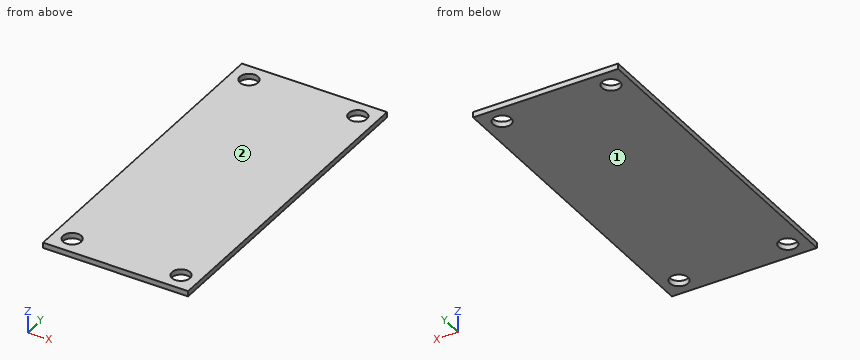
from build123d import *

# Parameters (mm, degrees)
SKETCH1_W           = 40
SKETCH1_H           = 41
BOSS_EXTRUDE1_DEPTH = 1.5
SKETCH2_R           = 2.5
CUT_EXTRUDE1_DEPTH  = 270.746640387


with BuildPart() as part:
    # Sketch1 → Boss-Extrude1 (new body)
    with BuildSketch(Plane.XY):
        Polygon((10, 269), (-10, 269), (-20, 269), (-20, 261), (-20, 220), (20, 220), (20, 261), (20, 269), align=None)
        with Locations((0, 199.5)):
            Rectangle(SKETCH1_W, SKETCH1_H)
    extrude(amount=BOSS_EXTRUDE1_DEPTH)

    # Sketch2 → Cut-Extrude1 (cut, through all)
    with BuildSketch(Plane.XY.offset(1.5)):
        with Locations((15, 264)):
            Circle(SKETCH2_R)
        with Locations(Location((15, 184, 0), (0, 0, 180))):
            Circle(SKETCH2_R)
        with Locations((-15, 184)):
            Circle(SKETCH2_R)
        with Locations(Location((-15, 264, 0), (0, 0, 180))):
            Circle(SKETCH2_R)
    extrude(amount=-CUT_EXTRUDE1_DEPTH, mode=Mode.SUBTRACT)


solid = part.part
The listing builds one solid part. Answer for the finished solid, in the listing's coordinates (mm). Face numbers are marked on the shaded views. Coordinates: 2 decimals unless noted, no trailing zeros. Order: outer loops, then holes, each group sorted by start corner. A loop starts at its lowest first (then second) coordinate and runs counter-clockwise, first axis right, second up.
Q1. For a pull along Z with two mould halves and no side action, classify the marked faces 1 and 2 as pulls with the +Z half, pulls with the -Z half, needs draft (parallel to the pull), parting line crosses it, or undercut.
Q2. A cutting plane is placed at A-A, the plane x = 15. Write down the section's boundary in (y, z).
Q3. A cutting plane is placed at C-C, the plane z = 0.75. Write down the section's boundary in (x, y), and give its area (3 significant figures).
Q4. Consider line 1 (Y direction, x = -15, z = 1); line 2 (X direction, y = 184, z = 0.45); line 3 (X direction, y = 262.5, z = 0.2). Determine where each line is inside the solid, lowest interval first.
Q5. A cutting plane is placed at B-B, the plane y = 184. Write down the section's boundary in (x, z), and give its area (3 significant figures).
Q6. Given P1, Ø6.5, axis at x = -15, y = 184, coming from the +Z side, flat-ended and moving along its own axis, determine where the tip first touches the part or whether it passes through.
Answers follow:
1. face 1: pulls with the -Z half
1. face 2: pulls with the +Z half
2. outline: (179, 0) - (181.5, 0) - (181.5, 1.5) - (179, 1.5) - close; (186.5, 0) - (261.5, 0) - (261.5, 1.5) - (186.5, 1.5) - close; (266.5, 0) - (269, 0) - (269, 1.5) - (266.5, 1.5) - close
3. outline: (-20, 179) - (20, 179) - (20, 269) - (-20, 269) - close; hole circle Ø5 at (-15, 184); hole circle Ø5 at (-15, 264); hole circle Ø5 at (15, 184); hole circle Ø5 at (15, 264)
3. area: 3,520 mm2
4. line 1: y = 179 to 181.5, 186.5 to 261.5, 266.5 to 269
4. line 2: x = -20 to -17.5, -12.5 to 12.5, 17.5 to 20
4. line 3: x = -20 to -17, -13 to 13, 17 to 20
5. outline: (-20, 0) - (-17.5, 0) - (-17.5, 1.5) - (-20, 1.5) - close; (-12.5, 0) - (12.5, 0) - (12.5, 1.5) - (-12.5, 1.5) - close; (17.5, 0) - (20, 0) - (20, 1.5) - (17.5, 1.5) - close
5. area: 45.0 mm2
6. P1: stops at z = 1.5
